Geometry check sheet. Reference: drawing and pictorial views, mm from the part's lowest x, y, z. A direction names the side the tool comes from. Give positions to 0.01 mm unless a question says otherwise; leave off trailing zeros. Loops run counter-clockwise (first coordinate to the right, second up) from the corner with the lowest first, then second, coordinate; pieces in that order, holes last. Notation, with made-up numbers: (19, 26.25) - (63, 26.25) arc R7 ccw to (63, 33.25) - close; hole circle Ø4 at (81, -34). An arc over 180 degrees is marked (long way). Answer in a Markdown table with one row per item. Add a question column.
(1) Thickness scan on L1, parallel to Y at x = 10, z = 30; L2, parallel to X at y = 11, z = 49 (1 decimal); L3, parallel to Z at x = 18.25, y = 15.5. Record the ranges inside material, lowest first.
(2) Go/stop test with flat-tipped pins: P1, Ø2, axis at y = 15, z = 78, coming from the +X side; P2, Ø8, axis at x = 4.5, z = 120.5, coming from the +Y side (1 decimal); P3, Ø3, axis at x = 16, y = 16, coming from the -Z side; P4, Ø2, axis at x = 5.5, z = 54, coming from the -Y side (1 decimal). Record where each tip stops, or that it passes through.
(3) Set-up check for the marked faces 1 and 2: record each of +Z, -Z, +X, -X, +Y, -Y from which the full face is reachable in a straight line by a thin tool's end or side.
(4) Sectioned sample at D-D on y = 2. Enter the section's corners in (x, z).
(5) Sectioned sample at B-B on y = 13.75. Enter the section's corners in (x, z), then the cut area to 3 significant figures.
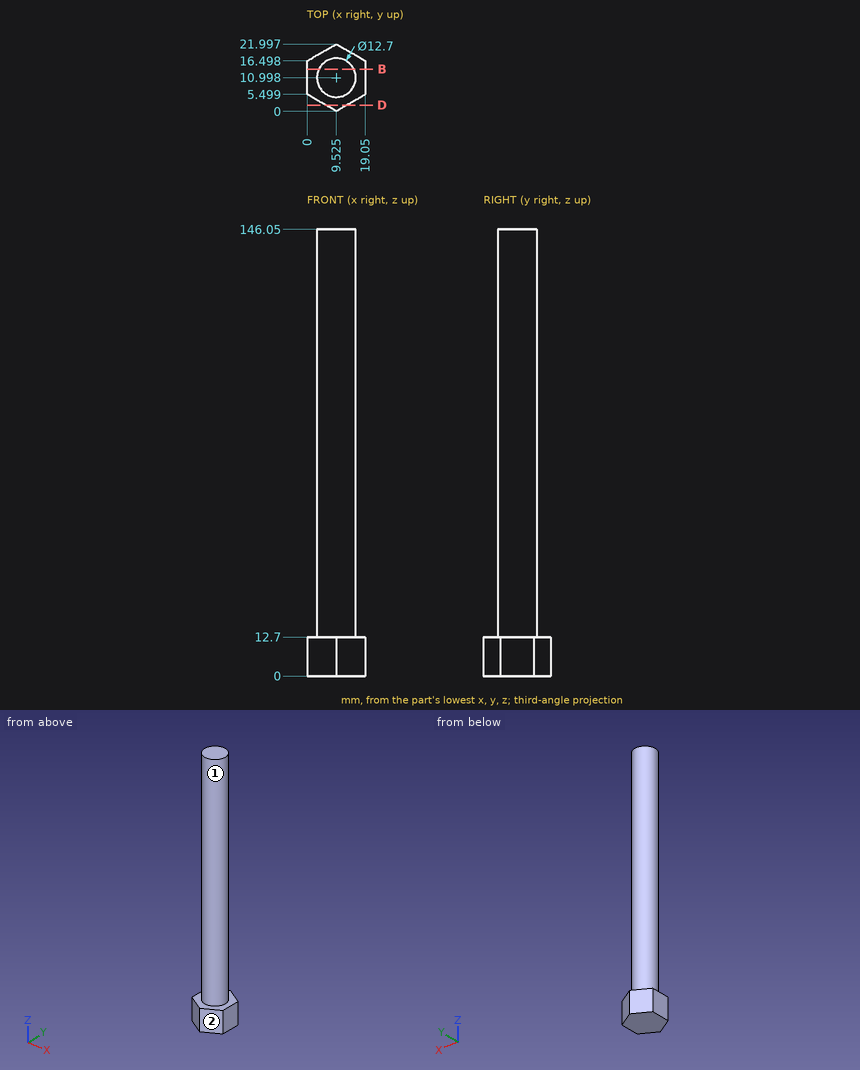
Reply:
| question | item | result |
|---|---|---|
| 1 | L1 | 4.67 to 17.33 |
| 1 | L2 | 3.2 to 15.9 |
| 1 | L3 | 0 to 12.7 |
| 2 | P1 | x = 15.12 |
| 2 | P2 | y = 17.3 |
| 2 | P3 | z = 0 |
| 2 | P4 | y = 5.4 |
| 3 | face 1 | +Z |
| 3 | face 2 | +Z, -Z, +X, -Y |
| 4 | outline | (6.06, 0) - (12.99, 0) - (12.99, 12.7) - (6.06, 12.7) - close |
| 5 | outline | (0, 0) - (19.05, 0) - (19.05, 12.7) - (15.25, 12.7) - (15.25, 146.05) - (3.8, 146.05) - (3.8, 12.7) - (0, 12.7) - close |
| 5 | area | 1,770 mm^2 |
